```python
from build123d import *

# Parameters (mm, degrees)
BOSS_EXTRUDE1_DEPTH                      = 3
BOSS_EXTRUDE2_START                      = 22
BOSS_EXTRUDE2_DEPTH                      = 3
SKETCH3_W                                = 1.5
SKETCH3_H                                = 28
F_3_0MM_CLEARANCE_DOWEL_HOLE1_AT_2_COUNT = 2
F_3_0MM_CLEARANCE_DOWEL_HOLE1_AT_2_PITCH = 28.1
SKETCH5_W                                = 43.073811931
SKETCH5_H                                = 3.925670489
BOSS_EXTRUDE3_DEPTH                      = 22
SKETCH6_W                                = 23
SKETCH6_H                                = 9.5
CUT_EXTRUDE1_DEPTH                       = 10
F_2_CLEARANCE_HOLE1_D                    = 2.4384


with BuildPart() as part:
    # Sketch1 → Boss-Extrude1 (new body)
    with BuildSketch(Plane(origin=(0, 0, 0), x_dir=(1, 0, 0), z_dir=(0, 1, 0))):
        with BuildLine():
            Line((-4.577926811, 9.356292891), (42.056666031, -6.499468675))
            ThreePointArc((42.056666031, -6.499468675), (42.793295664, -7.04620955), (43.073811931, -7.919627792))
            Line((43.073811931, -7.919627792), (43.073811931, -11.845298281))
            Line((43.073811931, -11.845298281), (0, -11.845298281))
            Line((0, -11.845298281), (0, 0.154701719))
            Line((0, 0.154701719), (-36.926188069, 0.154701719))
            Line((-36.926188069, 0.154701719), (-36.926188069, 10.154701719))
            Line((-36.926188069, 10.154701719), (-9.406467809, 10.154701719))
            ThreePointArc((-9.406467809, 10.154701719), (-6.959415254, 9.953753506), (-4.577926811, 9.356292891))
        make_face()
    extrude(amount=-BOSS_EXTRUDE1_DEPTH)


with BuildPart() as body_2:
    # Sketch1<2> → Boss-Extrude2 (new body)
    with BuildSketch(Plane(origin=(0, 0, 0), x_dir=(1, 0, 0), z_dir=(0, 1, 0)).offset(BOSS_EXTRUDE2_START)):
        with BuildLine():
            Line((-4.577926811, 9.356292891), (42.056666031, -6.499468675))
            ThreePointArc((42.056666031, -6.499468675), (42.793295664, -7.04620955), (43.073811931, -7.919627792))
            Line((43.073811931, -7.919627792), (43.073811931, -11.845298281))
            Line((43.073811931, -11.845298281), (0, -11.845298281))
            Line((0, -11.845298281), (0, 0.154701719))
            Line((0, 0.154701719), (-36.926188069, 0.154701719))
            Line((-36.926188069, 0.154701719), (-36.926188069, 10.154701719))
            Line((-36.926188069, 10.154701719), (-9.406467809, 10.154701719))
            ThreePointArc((-9.406467809, 10.154701719), (-6.959415254, 9.953753506), (-4.577926811, 9.356292891))
        make_face()
    extrude(amount=BOSS_EXTRUDE2_DEPTH)


with BuildPart() as f_3_0mm_clearance_dowel_hole1_tool:
    # Sketch3 → Ø3.0mm Clearance Dowel Hole1 (revolve)
    with BuildSketch(Plane(origin=(-33.926188069, -3, -5.154701719), x_dir=(0, 0, -1), z_dir=(1, 0, 0))):
        with Locations((0.75, 14)):
            Rectangle(SKETCH3_W, SKETCH3_H)
    f_3_0mm_clearance_dowel_hole1 = revolve(axis=Axis((-33.926188069, -9.35, -5.154701719), (0, 1, 0)))


with BuildPart() as part_1:
    add(part.part)

    # Ø3.0mm Clearance Dowel Hole1: cut by f_3_0mm_clearance_dowel_hole1_tool
    add(f_3_0mm_clearance_dowel_hole1_tool.part, mode=Mode.SUBTRACT)


with BuildPart() as body_2_1:
    add(body_2.part)

    # Ø3.0mm Clearance Dowel Hole1: cut by f_3_0mm_clearance_dowel_hole1_tool
    add(f_3_0mm_clearance_dowel_hole1_tool.part, mode=Mode.SUBTRACT)


with BuildPart() as f_3_0mm_clearance_dowel_hole1_at_2_tool:
    # Ø3.0mm Clearance Dowel Hole1 at 2: Ø3.0mm Clearance Dowel Hole1 ×2
    with Locations(*[(i * F_3_0MM_CLEARANCE_DOWEL_HOLE1_AT_2_PITCH, 0, 0) for i in range(1, F_3_0MM_CLEARANCE_DOWEL_HOLE1_AT_2_COUNT)]):
        add(f_3_0mm_clearance_dowel_hole1)


with BuildPart() as part_2:
    add(part_1.part)

    # Ø3.0mm Clearance Dowel Hole1 at 2: cut by f_3_0mm_clearance_dowel_hole1_at_2_tool
    add(f_3_0mm_clearance_dowel_hole1_at_2_tool.part, mode=Mode.SUBTRACT)



with BuildPart() as body_2_2:
    add(body_2_1.part)

    # Ø3.0mm Clearance Dowel Hole1 at 2: cut by f_3_0mm_clearance_dowel_hole1_at_2_tool
    add(f_3_0mm_clearance_dowel_hole1_at_2_tool.part, mode=Mode.SUBTRACT)


with BuildPart() as part_3:
    add(part_2.part)

    add(body_2_2.part)  # Boss-Extrude3 merges body 2
    # Sketch5 → Boss-Extrude3 (add)
    with BuildSketch(Plane(origin=(0, 0, 0), x_dir=(1, 0, 0), z_dir=(0, 1, 0))):
        with Locations((21.536905966, -9.882463037)):
            Rectangle(SKETCH5_W, SKETCH5_H)
    extrude(amount=BOSS_EXTRUDE3_DEPTH)

    # Sketch6 → Cut-Extrude1 (cut)
    with BuildSketch(Plane(origin=(0, 25, 0), x_dir=(1, 0, 0), z_dir=(0, 1, 0))):
        with Locations((21.5, -3.165298281)):
            Rectangle(SKETCH6_W, SKETCH6_H)
    extrude(amount=-CUT_EXTRUDE1_DEPTH, mode=Mode.SUBTRACT)

    # #2 Clearance Hole1 (through all)
    with Locations(Plane.XY.offset(11.845298281)):
        with Locations((16.75, 19), (26.25, 19)):
            Hole(F_2_CLEARANCE_HOLE1_D / 2)


solid = part_3.part
```
Can you work these out from the model? Positions are in its coordinate system, mm. A direction names the side the tool comes from. Round coordinates to 2 decimals unless told otherwise and drop trailing zeros. Loops run counter-clockwise (first coordinate to the right, second up) from the corner with the lowest first, then second, coordinate; pieces in that order, holes last.
Item 1: Suppose I cut it at D-D, the plane z = -4.5. Write out the boundary of the cut face in (x, y).
Item 2: Suppose I cut it at A-A, the plane y = 19. Write out the boundary of the cut face in (x, z), then the cut area to 3 significant figures.
Item 3: If we mould it in two halves opening along Z, with no side actions, what happens to faces 4 (the flat face through (6.691, 23.479, -5.525)), 5 (the flat face through (21, 24, 7.915)), 6 (the flat face through (33, 24, 6)), 7 (the cylindrical face through (-32.46, 23.52, -4.83))? For each: +Z half, -Z half, draft (parallel to the pull), parting line (faces both ways), or undercut.
Item 4: Will these pins go through, and if not, where does the flat tip stop? pin 1 Ø0.9 at (x, y) = (-18.5, -1.5) entering from +Z; pin 2 Ø4 at (x, y) = (32, 18) entering from -Z; pin 3 Ø1.5 at (x, y) = (18.5, 23.5) entering from -Z.
Item 5: Which directions (+Z, -Z, +X, -X, +Y, -Y) give clear straight access to the entire face, cutting with the end or side of a thin tool? Please do faces 1 (the flat face through (21, 11, 7.92)), 2 (the flat face through (-18, 23, -0.155)), 3 (the flat face through (-36.926, -1, -5)).
Item 6: Please list where these lines run through material, in increasing order: L1, parallel to Y at x = 16.75, z = 9.55; L2, parallel to Z at x = -16, y = 22.5; L3, parallel to Y at x = -31.5, z = -1.
Item 7: Suppose I cut it at B-B, the plane x = -18. Write out the boundary of the cut face in (y, z), then the cut area to 3 significant figures.
Item 8: Suppose I cut it at C-C, the plane x = 16.75. State how many separate pieces and enclosed holes the cut face has, then the cut area to 3 significant figures.
Reported:
1. outline: (-36.93, -3) - (-35.28, -3) - (-35.28, 0) - (-36.93, 0) - close; (-36.93, 22) - (-35.28, 22) - (-35.28, 25) - (-36.93, 25) - close; (-32.58, -3) - (-7.18, -3) - (-7.18, 0) - (-32.58, 0) - close; (-32.58, 22) - (-7.18, 22) - (-7.18, 25) - (-32.58, 25) - close; (-4.48, -3) - (9.71, -3) - (9.71, 0) - (-4.48, 0) - close; (-4.48, 22) - (9.71, 22) - (9.71, 25) - (-4.48, 25) - close
2. outline: (0, 7.92) - (15.53, 7.92) - (15.53, 11.85) - (0, 11.85) - close; (17.97, 7.92) - (25.03, 7.92) - (25.03, 11.85) - (17.97, 11.85) - close; (27.47, 7.92) - (43.07, 7.92) - (43.07, 11.85) - (27.47, 11.85) - close
2. area: 150 mm2
3. face 4: -Z half
3. face 5: undercut
3. face 6: draft
3. face 7: undercut
4. pin 1: stops at z = -0.15
4. pin 2: stops at z = 7.92
4. pin 3: stops at z = -1.76
5. face 1: -Z, +X, -X
5. face 2: +Z, -X, +Y, -Y
5. face 3: +Z, -Z, -X, +Y, -Y
6. L1: y = -3 to 17.78, 20.22 to 25
6. L2: z = -10.15 to -0.15
6. L3: y = -3 to 0, 22 to 25
7. outline: (-3, -10.15) - (0, -10.15) - (0, -0.15) - (-3, -0.15) - close; (22, -10.15) - (25, -10.15) - (25, -0.15) - (22, -0.15) - close
7. area: 60.0 mm2
8. separate pieces: 3
8. enclosed holes: 0
8. area: 132 mm2
